from build123d import *

# Parameters (mm, degrees)
BOSS_EXTRUDE1_DEPTH = 0.5
FILLET1_R           = 10
SKETCH27_R          = 4.5
CUT_EXTRUDE9_DEPTH  = 104.078853311
CUT_EXTRUDE17_DEPTH = 104.078853311


with BuildPart() as part:
    # Sketch1 → Boss-Extrude1 (new body)
    with BuildSketch(Plane(origin=(0, 0, 0), x_dir=(1, 0, 0), z_dir=(0, 1, 0))):
        with BuildLine():
            Line((-63, 65), (46.636895265, 65))
            ThreePointArc((46.636895265, 65), (80, 0), (46.636895265, -65))
            Line((46.636895265, -65), (-63, -65))
            Line((-63, -65), (-63, 65))
        make_face()
    extrude(amount=BOSS_EXTRUDE1_DEPTH)

    # Fillet1
    fillet1_edges = [part.edges().sort_by_distance(p)[0] for p in [
        (-63, 0.25, -65),
        (-63, 0.25, 65),
    ]]
    fillet(fillet1_edges, radius=FILLET1_R)

    # Sketch27 → Cut-Extrude9 (cut, through all)
    with BuildSketch(Plane(origin=(0, 0.5, 0), x_dir=(1, 0, 0), z_dir=(0, 1, 0))):
        with Locations(Location((-49.497474683, -49.497474683, 0), (0, 0, 270))):
            Circle(SKETCH27_R)
        with Locations(Location((49.497474683, -49.497474683, 0), (0, 0, 270))):
            Circle(SKETCH27_R)
        with Locations(Location((49.497474683, 49.497474683, 0), (0, 0, 270))):
            Circle(SKETCH27_R)
        with Locations(Location((-49.497474683, 49.497474683, 0), (0, 0, 270))):
            Circle(SKETCH27_R)
    extrude(amount=-CUT_EXTRUDE9_DEPTH, mode=Mode.SUBTRACT)

    # Sketch44 → Cut-Extrude17 (cut, through all)
    with BuildSketch(Plane(origin=(0, 0.5, 0), x_dir=(1, 0, 0), z_dir=(0, 1, 0))):
        with BuildLine():
            Line((47.997474683, 38.997474683), (62.89035672, 38.997474683))
            ThreePointArc((62.89035672, 38.997474683), (74, 0), (62.89035672, -38.997474683))
            Line((62.89035672, -38.997474683), (47.997474683, -38.997474683))
            ThreePointArc((47.997474683, -38.997474683), (41.633513652, -41.633513652), (38.997474683, -47.997474683))
            Line((38.997474683, -47.997474683), (38.997474683, -50))
            ThreePointArc((38.997474683, -50), (36.361435714, -56.363961031), (29.997474683, -59))
            Line((29.997474683, -59), (-29.997474683, -59))
            ThreePointArc((-29.997474683, -59), (-36.361435714, -56.363961031), (-38.997474683, -50))
            Line((-38.997474683, -50), (-38.997474683, -47.997474683))
            ThreePointArc((-38.997474683, -47.997474683), (-41.633513652, -41.633513652), (-47.997474683, -38.997474683))
            Line((-47.997474683, -38.997474683), (-57, -38.997474683))
            Line((-57, -38.997474683), (-57, 38.997474683))
            Line((-57, 38.997474683), (-47.997474683, 38.997474683))
            ThreePointArc((-47.997474683, 38.997474683), (-41.633513652, 41.633513652), (-38.997474683, 47.997474683))
            Line((-38.997474683, 47.997474683), (-38.997474683, 50))
            ThreePointArc((-38.997474683, 50), (-36.361435714, 56.363961031), (-29.997474683, 59))
            Line((-29.997474683, 59), (29.997474683, 59))
            ThreePointArc((29.997474683, 59), (36.361435714, 56.363961031), (38.997474683, 50))
            Line((38.997474683, 50), (38.997474683, 47.997474683))
            ThreePointArc((38.997474683, 47.997474683), (41.633513652, 41.633513652), (47.997474683, 38.997474683))
        make_face()
    extrude(amount=-CUT_EXTRUDE17_DEPTH, mode=Mode.SUBTRACT)


solid = part.part
Geometry: final body of the model. Coordinates: model frame, mm. A direction names the side the tool comes from. Round coordinates to 2 decimals unless told otherwise and drop trailing zeros. Order: outer loops, then holes, each group sorted by start corner. A loop starts at its lowest first (then second) coordinate and runs counter-clockwise, first axis right, second up. Notation, with made-up numbers: (-16.75, -16) -> (39.25, -16) arc R28 cw to (39.25, 17) -> close; hole circle Ø1 at (60, -3). An arc over 180 degrees is marked (long way). Put each result on its own line as item: value. Start each with the question number.
Q1. Section B-B on z = 17. Return the cut outline in (x, y), and give its area (3 significant figures).
Q2. Reachability of faces 5 (the flat face through (41, 0.5, -44)), 6 (the cylindrical face through (-41.704, 0.254, -41.564)) from +Z, -Z, +X, -X, +Y, -Y: full face, straight path, thin tool, end or side. Return the list, or none.
Q3. Section A-A on x = -22. Return the cut outline in (y, z).
Q4. Line query: probe 1 along Z at (x, y) = (8, 0.3); probe 2 along X at (y, z) = (0.25, 42.5); probe 3 along X at (y, z) = (0.1, 47). Output: solid intervals per line, ascending.
Q5. First-contact query: pin 1 (7 mm diameter, centred on x = -49.5, z = -49.5, fed in from +Y). Flat tip, straight axial feed; report the tip coordinate or a pass-through.
Q6. Pull-direction query (X, two-part tool) for faces 1 (the flat face through (41, 0, -44)), 2 (the cylindrical face through (-41.564, 0.254, 41.704)), 3 (the cylindrical face through (-59.99, 0.25, 62.15)), 4 (the cylindrical face through (79.993, 0.246, -1.062)); classes: +X half, -X half, draft (parallel to the pull), parting line (faces both ways), or undercut.
Q7. Section C-C on y = 0.1. Give the number of separate pieces and of enclosed holes in the cut face, and give its area (3 significant figures).
Ans:
1. outline: (-63, 0) -> (-57, 0) -> (-57, 0.5) -> (-63, 0.5) -> close; (72.02, 0) -> (78.17, 0) -> (78.17, 0.5) -> (72.02, 0.5) -> close
1. area: 6.08 mm2
2. face 5: +Z, -Z, +X, -X, +Y
2. face 6: +Y, -Y
3. outline: (0, -65) -> (0.5, -65) -> (0.5, -59) -> (0, -59) -> close; (0, 59) -> (0.5, 59) -> (0.5, 65) -> (0, 65) -> close
4. probe 1: z = -65 to -59, 59 to 65
4. probe 2: x = -63 to -40.87, 40.87 to 67.78
4. probe 3: x = -63 to -53.24, -45.75 to -39.05, 39.05 to 45.75, 53.24 to 64.74
5. pin 1: passes through
6. face 1: draft
6. face 2: undercut
6. face 3: -X half
6. face 4: +X half
7. separate pieces: 1
7. enclosed holes: 5
7. area: 3,940 mm2
